Autodesk Inventor part; units mm, degrees
ref_plane "YZ Plane" through (0, 0, 0) normal (1, 0, 0) x (0, 1, 0)
ref_plane "XZ Plane" through (0, 0, 0) normal (0, 1, 0) x (-1, 0, 0)
ref_plane "XY Plane" through (0, 0, 0) normal (0, 0, 1) x (1, 0, 0)
sketch "Sketch1" plane through (0, 0, 0) normal (0, 0, 1) x (1, 0, 0)
  line L0 (0, 0) -> (6, 0)
  line L1 (6, 0) -> (6, 7.5)
  line L2 (6, 7.5) -> (0, 7.5)
  line L3 (0, 7.5) -> (0, 0)
  line L4 (6, 0) -> (10, 0)
  line L5 (10, 0) -> (10, 8.5)
  line L6 (10, 8.5) -> (6, 8.5)
  line L7 (6, 8.5) -> (6, 0)
  dimension "d0" = 15
  dimension "d1" = 17
  dimension "d2" = 6
  dimension "d3" = 10
revolve "Revolution1" add sketch "Sketch1" angle 360 about axis through (0, 0, 0) along (1, 0, 0)
fillet "Fillet1" radius 1.5 1 edges at (6, -8.5, 0)
hole "Hole1" at (10, 0, 0) direction (-1, 0, 0) diameter 13 end through all
properties part number "405-03" material "Steel, Mild"
Here's how the part is built. I have some questions about the finished solid (model axes, mm). A direction names the side the tool comes from. Coordinates: 2 decimals unless noted, no trailing zeros. Write each loop counter-clockwise with the first axis right and the second up, starting at its lowest first coordinate (ties: lowest second). Pieces come first, ordered by that corner, then holes.
1) If we section it at C-C (x = 9.5): List the corners of the cut face in (y, z) for me.
Filled in:
outline: circle Ø17 at (0, 0); hole circle Ø13 at (0, 0)
2) Which directions (+Z, -Z, +X, -X, +Y, -Y) give clear straight access to the entire face, cutting with the end or side of a thin tool? Please do faces 4 (the face through (2.958, -7.493, -0.33)), 5 (the face through (0, -6, 3)).
Filled in:
face 4: -X
face 5: +Z, -Z, -X, +Y, -Y
3) I'm going to push flat-ended pins straight in: pin 1 (4 mm diameter, centred on x = 4.5, y = -4, fed in from +Z); pin 2 (8 mm diameter, centred on y = 5, z = 2.5, fed in from -X); pin 3 (5 mm diameter, centred on x = 6.5, z = 3, fed in from -Y); pin 4 (1.5 mm diameter, centred on x = 8.5, y = 6.5, fed in from -Z). Where does each tip first touch, or does it pass through?
Filled in:
pin 1: stops at z = 7.38
pin 2: stops at x = 0
pin 3: stops at y = -8.47
pin 4: stops at z = -6.26
4) If we section it at A-A (y = 0): List the corners of the cut face in (x, z) for me, plus the area to 3 significant figures.
Filled in:
outline: (0, -7.5) - (6, -7.5) arc R1.5 ccw to (7.41, -8.5) - (10, -8.5) - (10, -6.5) - (0, -6.5) - close; (0, 6.5) - (10, 6.5) - (10, 8.5) - (7.41, 8.5) arc R1.5 ccw to (6, 7.5) - (0, 7.5) - close
area: 27.2 mm2
5) If we section it at D-D (x = 1): List the corners of the cut face in (y, z) for me, plus the area to 3 significant figures.
Filled in:
outline: circle Ø15 at (0, 0); hole circle Ø13 at (0, 0)
area: 44.0 mm2
6) Thinking about a two-plate mould opening in Z: for faces 1 (the face through (10, 4.4, -5)), 2 (the face through (8.689, 4.57, -7.167)), 3 (the face through (4.93, 3.955, 5.158)), which applies, +Z half, -Z half, draft (parallel to the pull), parting line (faces both ways), or undercut?
Filled in:
face 1: draft
face 2: parting line
face 3: undercut
7) If I drill on line 1 (Z direction, x = 3, y = 0); line 2 (Y direction, x = 6.5, z = -3.5); line 3 (Z direction, x = 7.25, y = 0.5), over which ranges is the centre line in solid material (lowest first)?
Filled in:
line 1: z = -7.5 to -6.5, 6.5 to 7.5
line 2: y = -7.4 to -5.48, 5.48 to 7.4
line 3: z = -8.48 to -6.48, 6.48 to 8.48
